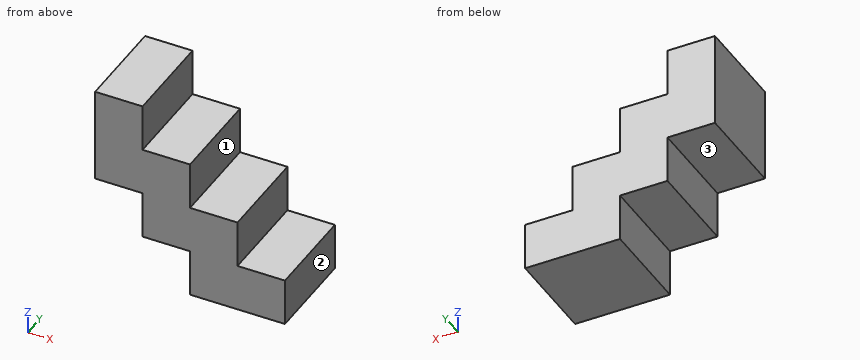
```python
from build123d import *

# Parameters (mm, degrees)
F0_W      = 152.4
F0_H      = 152.4
F1_DEPTH  = 152.4
F2_W      = 76.2
F2_H      = 76.2
F3_DEPTH  = 271.78
F4_W      = 152.4
F4_H      = 76.2
F5_DEPTH  = 76.2
F6_W      = 76.2
F6_H      = 152.4
F7_DEPTH  = 76.2
F8_W      = 76.2
F8_H      = 152.4
F9_DEPTH  = 76.2
F10_W     = 152.4
F10_H     = 76.2
F11_DEPTH = 76.2


with BuildPart() as f1:
    # F0 (on Front) → F1 (new body)
    with BuildSketch(Plane.XZ):
        Rectangle(F0_W, F0_H)
    extrude(amount=F1_DEPTH)

    # F2 (on face) → F3 (cut)
    with BuildSketch(Plane.XZ.offset(152.4)):
        with Locations((38.1, 38.1)):
            Rectangle(F2_W, F2_H)
    extrude(amount=-F3_DEPTH, mode=Mode.SUBTRACT)

    # F4 (on face) → F5 (join, symmetric)
    with BuildSketch(Plane(origin=(-76.2, 0, 0), x_dir=(0, -1, 0), z_dir=(-1, 0, 0))):
        with Locations((76.2, 38.1)):
            Rectangle(F4_W, F4_H)
    extrude(amount=F5_DEPTH, both=True)

    # F6 (on face) → F7 (join)
    with BuildSketch(Plane(origin=(0, 0, -76.2), x_dir=(1, 0, 0), z_dir=(0, 0, -1))):
        with Locations((38.1, 76.2)):
            Rectangle(F6_W, F6_H)
    extrude(amount=F7_DEPTH)

    # F8 (on face) → F9 (join)
    with BuildSketch(Plane.XY.offset(76.2)):
        with Locations((-114.3, -76.2)):
            Rectangle(F8_W, F8_H)
    extrude(amount=F9_DEPTH)

    # F10 (on face) → F11 (join, symmetric)
    with BuildSketch(Plane.YZ.offset(76.2)):
        with Locations((-76.2, -114.3)):
            Rectangle(F10_W, F10_H)
    extrude(amount=F11_DEPTH, both=True)


solid = f1.part
```
Input: part model. Units: mm. Frame: model coordinates. Face numbers are marked on the shaded views. A direction names the side the tool comes from. Give positions to 0.01 mm unless a question says otherwise; leave off trailing zeros. Order: outer loops, then holes, each group sorted by start corner. A loop starts at its lowest first (then second) coordinate and runs counter-clockwise, first axis right, second up. Notation, with made-up numbers: (24, 73.5) -> (52, 73.5) arc R13 cw to (52, 77.5) -> close; hole circle Ø1 at (76, 5). An arc over 180 degrees is marked (long way). Write each question's results on one line, items separated by ' | '. Start each with the question number.
Item 1: Line query: line 1 (Z direction, x = -126.5, y = -125); line 2 (Z direction, x = 77.5, y = -53). Output: solid intervals per line, ascending.
Item 2: Cut plane A-A on y = -26. Return the cut outline in (x, z).
Item 3: Set-up query: the marked faces 1, 2 and 3. Return all of +Z, -Z, +X, -X, +Y, -Y with unobstructed straight access to the full face (end or side cutting, diameter ignored); none if empty.
Item 4: Cut plane B-B on x = -56. Return the cut outline in (y, z), then the cut area to 3 significant figures.
Item 5: Cut plane C-C on z = 122. Return the cut outline in (x, y).
Item 6: Contact query for flat-ended pins moving along their axis: P1, Ø23, axis at x = -44.5, y = -59, coming from the +Z side; P2, Ø23, axis at x = 46, y = -45, coming from the +Z side; P3, Ø23, axis at x = -49, y = -68.5, coming from the -Z side. Output: stop coordinate, or through.
Established:
1) line 1: 0 to 152.4 | line 2: -152.4 to -76.2
2) outline: (-152.4, 0) -> (-76.2, 0) -> (-76.2, -76.2) -> (0, -76.2) -> (0, -152.4) -> (152.4, -152.4) -> (152.4, -76.2) -> (76.2, -76.2) -> (76.2, 0) -> (0, 0) -> (0, 76.2) -> (-76.2, 76.2) -> (-76.2, 152.4) -> (-152.4, 152.4) -> close
3) face 1: +Z, +X, +Y, -Y | face 2: +Z, -Z, +X, +Y, -Y | face 3: -Z, -X, +Y, -Y
4) outline: (-152.4, -76.2) -> (0, -76.2) -> (0, 76.2) -> (-152.4, 76.2) -> close | area: 23,200 mm^2
5) outline: (-152.4, -152.4) -> (-76.2, -152.4) -> (-76.2, 0) -> (-152.4, 0) -> close
6) P1: z = 76.2 | P2: z = 0 | P3: z = -76.2
